from build123d import *

# Parameters (mm, degrees)
BOSS_EXTRUDE1_DEPTH     = 156
FILLET1_R               = 6
SKETCH2_R               = 2.05
CUT_EXTRUDE1_DEPTH      = 157.511980372
LPATTERN1_COUNT         = 9
LPATTERN1_PITCH         = 8
MIRROR1_COPY_1_SKETCH_R = 2.05
MIRROR1_COPY_1_DEPTH    = 157.511980372
MIRROR1_COPY_2_SKETCH_R = 2.05
MIRROR1_COPY_2_DEPTH    = 157.511980372
MIRROR1_COPY_3_SKETCH_R = 2.05
MIRROR1_COPY_3_DEPTH    = 157.511980372
MIRROR1_COPY_4_SKETCH_R = 2.05
MIRROR1_COPY_4_DEPTH    = 157.511980372
MIRROR1_COPY_5_SKETCH_R = 2.05
MIRROR1_COPY_5_DEPTH    = 157.511980372
MIRROR1_COPY_6_SKETCH_R = 2.05
MIRROR1_COPY_6_DEPTH    = 157.511980372


with BuildPart() as part:
    # Sketch1 → Boss-Extrude1 (new body)
    with BuildSketch(Plane.XY):
        Polygon((0, 0), (4, 0), (4, 2), (3, 2), (3, 10), (4, 10), (4, 12), (0, 12), align=None)
    extrude(amount=-BOSS_EXTRUDE1_DEPTH)

    # Fillet1
    fillet1_edges = [part.edges().sort_by_distance(p)[0] for p in [
        (2, 12, 0),
        (2, 0, 0),
        (2, 0, -156),
        (2, 12, -156),
    ]]
    fillet(fillet1_edges, radius=FILLET1_R - 0.0001)  # a hair under: the kernel refuses the full size

    # Sketch2 → Cut-Extrude1 (cut, through all)
    with BuildSketch(Plane.ZY):
        with Locations(Location((-150, 6, 0), (0, 0, 270))):
            Circle(SKETCH2_R)
    cut_extrude1 = extrude(amount=-CUT_EXTRUDE1_DEPTH, mode=Mode.SUBTRACT)

    # LPattern1: Cut-Extrude1 ×9, 2 skipped
    with Locations(*[(0, 0, i * LPATTERN1_PITCH) for i in range(1, LPATTERN1_COUNT) if i not in (5, 7)]):
        add(cut_extrude1, mode=Mode.SUBTRACT)

    # Mirror1: Cut-Extrude1 across plane
    add(cut_extrude1.mirror(Plane.XY.offset(-78)), mode=Mode.SUBTRACT)

    # Mirror1 copy 1 sketch → Mirror1 copy 1 (cut, through all)
    with BuildSketch(Plane(origin=(0, 0, -164), x_dir=(0, 0, -1), z_dir=(-1, 0, 0))):
        with Locations((-150, -6)):
            Circle(MIRROR1_COPY_1_SKETCH_R)
    extrude(amount=-MIRROR1_COPY_1_DEPTH, mode=Mode.SUBTRACT)

    # Mirror1 copy 2 sketch → Mirror1 copy 2 (cut, through all)
    with BuildSketch(Plane(origin=(0, 0, -172), x_dir=(0, 0, -1), z_dir=(-1, 0, 0))):
        with Locations((-150, -6)):
            Circle(MIRROR1_COPY_2_SKETCH_R)
    extrude(amount=-MIRROR1_COPY_2_DEPTH, mode=Mode.SUBTRACT)

    # Mirror1 copy 3 sketch → Mirror1 copy 3 (cut, through all)
    with BuildSketch(Plane(origin=(0, 0, -180), x_dir=(0, 0, -1), z_dir=(-1, 0, 0))):
        with Locations((-150, -6)):
            Circle(MIRROR1_COPY_3_SKETCH_R)
    extrude(amount=-MIRROR1_COPY_3_DEPTH, mode=Mode.SUBTRACT)

    # Mirror1 copy 4 sketch → Mirror1 copy 4 (cut, through all)
    with BuildSketch(Plane(origin=(0, 0, -188), x_dir=(0, 0, -1), z_dir=(-1, 0, 0))):
        with Locations((-150, -6)):
            Circle(MIRROR1_COPY_4_SKETCH_R)
    extrude(amount=-MIRROR1_COPY_4_DEPTH, mode=Mode.SUBTRACT)

    # Mirror1 copy 5 sketch → Mirror1 copy 5 (cut, through all)
    with BuildSketch(Plane(origin=(0, 0, -204), x_dir=(0, 0, -1), z_dir=(-1, 0, 0))):
        with Locations((-150, -6)):
            Circle(MIRROR1_COPY_5_SKETCH_R)
    extrude(amount=-MIRROR1_COPY_5_DEPTH, mode=Mode.SUBTRACT)

    # Mirror1 copy 6 sketch → Mirror1 copy 6 (cut, through all)
    with BuildSketch(Plane(origin=(0, 0, -220), x_dir=(0, 0, -1), z_dir=(-1, 0, 0))):
        with Locations((-150, -6)):
            Circle(MIRROR1_COPY_6_SKETCH_R)
    extrude(amount=-MIRROR1_COPY_6_DEPTH, mode=Mode.SUBTRACT)


solid = part.part
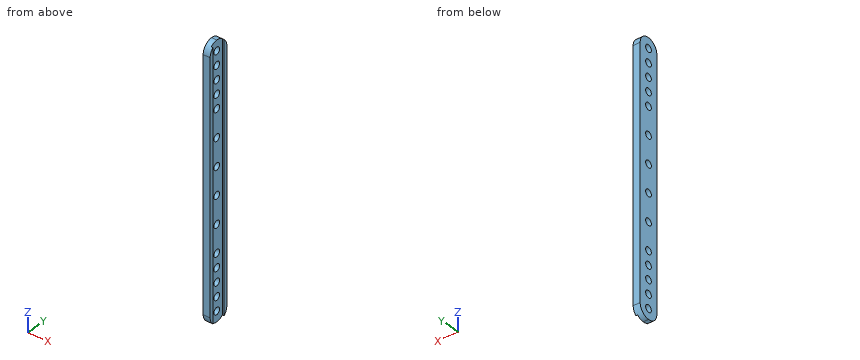
Could you check a few things on this model? Use its own coordinates, in mm. Round coordinates to 2 decimals unless told otherwise and drop trailing zeros. Order: outer loops, then holes, each group sorted by start corner. A loop starts at its lowest first (then second) coordinate and runs counter-clockwise, first axis right, second up.
(1) I'm going to push flat-ended pins straight in: pin 1 (6.5 mm diameter, centred on y = 6, z = -126, fed in from -X); pin 2 (5.5 mm diameter, centred on y = 6, z = -150, fed in from +X); pin 3 (1.5 mm diameter, centred on x = 0.5, y = 7, fed in from +Z). Where does each tip first touch, or does it pass through?
Response values:
pin 1: stops at x = 0
pin 2: stops at x = 3
pin 3: stops at z = -0.01
(2) Imagine slicing it at A-A (z = -30). Write out the boundary of the cut face in (x, y), plus the area to 3 significant figures.
Response values:
outline: (0, 0) - (4, 0) - (4, 2) - (3, 2) - (3, 3.95) - (0, 3.95) - close; (0, 8.05) - (3, 8.05) - (3, 10) - (4, 10) - (4, 12) - (0, 12) - close
area: 27.7 mm2
(3) Please list where these lines run through material, in increasing order: line 1 along Y through (x, z) = (0.6, -54); line 2 along X through (y, z) = (3, -63.5); line 3 along Y through (x, z) = (0.8, -127.5).
Response values:
line 1: y = 0 to 3.95, 8.05 to 12
line 2: x = 0 to 3
line 3: y = 0 to 4.6, 7.4 to 12
